Model file for the job. Use its own axes, mm. A direction names the side the tool comes from. Round coordinates to 2 decimals unless told otherwise and drop trailing zeros. Order: outer loops, then holes, each group sorted by start corner. A loop starts at its lowest first (then second) coordinate and runs counter-clockwise, first axis right, second up. Notation, with made-up numbers: (-7.75, 85) -> (20.25, 85) arc R17 cw to (20.25, 90) -> close; hole circle Ø4 at (34.25, -5). An arc over 180 degrees is marked (long way). Use CSV: the item, a comma, the result in double quotes.
```python
from build123d import *

# Parameters (mm, degrees)
F0_R            = 44.8437
F0_R_2          = 17.4625
F0_W            = 19.05
F0_H            = 6.35
F1_DEPTH        = 12.7
F2_DEPTH        = 6.35
F2_COPIES_COUNT = 4
F3_DEPTH        = 12.701
F3_COPIES_COUNT = 4


# Not quite as in the source:
# - a pattern or mirror of a feature is missing from the dataset's text; its kind, count and spacing are read off the source's solid


with BuildPart() as f1:
    # F0 (on Top) → F1 (new body)
    with BuildSketch(Plane.XY):
        with BuildLine():
            ThreePointArc((-9.525, 139.3749058296), (-95.3557746023, -102.0948884617), (139.7, 0))
            ThreePointArc((139.7, 0), (102.0948884617, 95.3557746023), (9.525, 139.3749058296))
            Line((9.525, 139.3749058296), (9.525, 120.3249058296))
            Line((9.525, 120.3249058296), (9.525, 113.9749058296))
            Line((9.525, 113.9749058296), (-9.525, 113.9749058296))
            Line((-9.525, 113.9749058296), (-9.525, 120.3249058296))
            Line((-9.525, 120.3249058296), (-9.525, 139.3749058296))
        make_face()
        Circle(F0_R, mode=Mode.SUBTRACT)
        with Locations((101.4398184138, 36.921074472)):
            Circle(F0_R_2, mode=Mode.SUBTRACT)
        with Locations((36.921074472, 101.4398184138)):
            Circle(F0_R_2, mode=Mode.SUBTRACT)
        with Locations((76.3321770291, 76.3321770291)):
            Circle(F0_R_2, mode=Mode.SUBTRACT)
        with BuildLine():
            Line((9.525, 120.3249058296), (9.525, 139.3749058296))
            ThreePointArc((9.525, 139.3749058296), (0, 139.7), (-9.525, 139.3749058296))
            Line((-9.525, 139.3749058296), (-9.525, 120.3249058296))
            Line((-9.525, 120.3249058296), (9.525, 120.3249058296))
        make_face()
        with Locations((36.921074472, 101.4398184138)):
            Circle(F0_R_2)
        with Locations((76.3321770291, 76.3321770291)):
            Circle(F0_R_2)
        with Locations((101.4398184138, 36.921074472)):
            Circle(F0_R_2)
        with Locations((0, 117.1499058296)):
            Rectangle(F0_W, F0_H)
        Circle(F0_R)
    extrude(amount=-F1_DEPTH)

    # F0 (on Top) → F2 (cut)
    with BuildSketch(Plane.XY):
        with Locations((36.921074472, 101.4398184138)):
            Circle(F0_R_2)
        with Locations((76.3321770291, 76.3321770291)):
            Circle(F0_R_2)
        with Locations((101.4398184138, 36.921074472)):
            Circle(F0_R_2)
    f2 = extrude(amount=-F2_DEPTH, mode=Mode.SUBTRACT)

    # F2_copies: F2 ×4 about axis
    f2_copies_axis = Axis((0, 0, 0), (0, 0, 1))
    for i in range(1, F2_COPIES_COUNT):
        add(f2.rotate(f2_copies_axis, i * 360 / F2_COPIES_COUNT), mode=Mode.SUBTRACT)

    # F0 (on Top) → F3 (cut, through all)
    with BuildSketch(Plane.XY):
        with BuildLine():
            Line((9.525, 120.3249058296), (9.525, 139.3749058296))
            ThreePointArc((9.525, 139.3749058296), (0, 139.7), (-9.525, 139.3749058296))
            Line((-9.525, 139.3749058296), (-9.525, 120.3249058296))
            Line((-9.525, 120.3249058296), (9.525, 120.3249058296))
        make_face()
    f3 = extrude(amount=-F3_DEPTH, mode=Mode.SUBTRACT)

    # F3_copies: F3 ×4 about axis
    f3_copies_axis = Axis((0, 0, 0), (0, 0, 1))
    for i in range(1, F3_COPIES_COUNT):
        add(f3.rotate(f3_copies_axis, i * 360 / F3_COPIES_COUNT), mode=Mode.SUBTRACT)


solid = f1.part
```
Q1. Cut at B-B (x = -32). Give the cut face in (y, z).
From the geometry:
outline,"(-135.99, -12.7) -> (135.99, -12.7) -> (135.99, 0) -> (118.19, 0) -> (118.19, -6.35) -> (84.69, -6.35) -> (84.69, 0) -> (-84.69, 0) -> (-84.69, -6.35) -> (-118.19, -6.35) -> (-118.19, 0) -> (-135.99, 0) -> close"
Q2. Cut at A-A (z = -2). State how many separate pieces and enclosed holes the cut face has, plus the area to 3 significant figures.
From the geometry:
separate pieces,"1"
enclosed holes,"12"
area,"48,300 mm²"
Q3. Which spindle directions (+Z, -Z, +X, -X, +Y, -Y) get a long thin tool onto all of the face, cutting with end or side? Do faces 1 (the flat face through (9.525, -130, -6)), 2 (the cylindrical face through (-99.77, -97.786, -6.261)), 3 (the flat face through (37, 102, -6.35)), 4 (the flat face through (9.525, 130, -6)). Say none if no direction does.
From the geometry:
face 1,"+Z, -Z, -Y"
face 2,"+Z, -Z, -X, -Y"
face 3,"+Z"
face 4,"+Z, -Z, +Y"
Q4. Cut at C-C (y = 89). Give the cut face in (x, z), plus the area to 3 significant figures.
From the geometry:
outline,"(-107.68, -12.7) -> (107.68, -12.7) -> (107.68, 0) -> (88.35, 0) -> (88.35, -6.35) -> (64.31, -6.35) -> (64.31, 0) -> (49.18, 0) -> (49.18, -6.35) -> (24.67, -6.35) -> (24.67, 0) -> (-24.67, 0) -> (-24.67, -6.35) -> (-49.18, -6.35) -> (-49.18, 0) -> (-64.31, 0) -> (-64.31, -6.35) -> (-88.35, -6.35) -> (-88.35, 0) -> (-107.68, 0) -> close"
area,"2,120 mm²"
Q5. Cut at D-D (y = -69.5). Give the cut face in (x, z), plus the area to 3 significant figures.
From the geometry:
outline,"(-121.19, -12.7) -> (121.19, -12.7) -> (121.19, 0) -> (92.4, 0) -> (92.4, -6.35) -> (60.26, -6.35) -> (60.26, 0) -> (-60.26, 0) -> (-60.26, -6.35) -> (-92.4, -6.35) -> (-92.4, 0) -> (-121.19, 0) -> close"
area,"2,670 mm²"
Q6. Mould opens along X. For faces 5 (the flat face through (120.325, 0, -6)), 6 (the flat face through (-76, -77, -6.35)), 7 (the flat face through (-2, 2, -12.7)), 8 (the cylindrical face through (-92.988, -81.577, -3.131)) say: +X half, -X half, draft (parallel to the pull), parting line (faces both ways), or undercut.
From the geometry:
face 5,"+X half"
face 6,"undercut"
face 7,"draft"
face 8,"undercut"
Q7. Pin check, flat tips, straight feed: pin 1 (1.5 mm diameter, centred on y = 60.5, z = -6, fed in from -X); pin 2 (4 mm diameter, centred on x = 128.5, z = -3.5, fed in from +Y); pin 3 (2 mm diameter, centred on x = -78, y = 65.5, fed in from +Z). Stop position of each tip, or through.
From the geometry:
pin 1,"stops at x = -126.28"
pin 2,"stops at y = 59.28"
pin 3,"stops at z = -6.35"
Q8. Probe line 1 along X through (y, z) = (43, -1.25); line 2 along Y through (x, z) = (111, -0.75); line 3 along X through (y, z) = (74.5, -2.5). List the from-to ranges inside material, lowest first.
From the geometry:
line 1,"x = -132.92 to -117.81, -85.07 to 85.07, 117.81 to 132.92"
line 2,"y = -84.82 to -51.53, -22.31 to 22.31, 51.53 to 84.82"
line 3,"x = -118.18 to -93.7, -58.97 to 58.97, 93.7 to 118.18"
